Verification items for the finished model (mm, model axes). Face numbers are marked on the shaded views. A direction names the side the tool comes from. Coordinates: 2 decimals unless noted, no trailing zeros. Write each loop counter-clockwise with the first axis right and the second up, starting at its lowest first coordinate (ties: lowest second). Pieces come first, ordered by that corner, then holes. Notation, with made-up numbers: M 45.25,71 L 66.25,71 A12 cw 66.25,88 Z; hole C -34,66.5 d1. An arc over 180 degrees is marked long. One line per item, written item: value.
```python
from build123d import *

# Parameters (mm, degrees)
SKETCH1_W           = 82
SKETCH1_H           = 31
BOSS_EXTRUDE2_DEPTH = 9.525
FILLET2_R           = 2
SKETCH2_R           = 8.119849814
CUT_EXTRUDE1_DEPTH  = 10.525
SKETCH3_W           = 9.5
SKETCH3_H           = 18
CUT_EXTRUDE2_DEPTH  = 10.525
SKETCH5_R           = 2.5
CUT_EXTRUDE4_DEPTH  = 30


with BuildPart() as part:
    # Sketch1 → Boss-Extrude2 (new body)
    with BuildSketch(Plane.XY):
        with Locations((0, 15.5)):
            Rectangle(SKETCH1_W, SKETCH1_H)
    extrude(amount=BOSS_EXTRUDE2_DEPTH)

    # Fillet2
    fillet2_edges = [part.edges().sort_by_distance(p)[0] for p in [
        (-41, 31, 4.7625),
        (41, 31, 4.7625),
        (41, 0, 4.7625),
        (-41, 0, 4.7625),
    ]]
    fillet(fillet2_edges, radius=FILLET2_R)

    # Sketch2 → Cut-Extrude1 (cut, through all)
    with BuildSketch(Plane.XY.offset(9.525)):
        with Locations((0, 15.5)):
            Circle(SKETCH2_R)
    extrude(amount=-CUT_EXTRUDE1_DEPTH, mode=Mode.SUBTRACT)

    # Sketch3 → Cut-Extrude2 (cut, through all)
    with BuildSketch(Plane(origin=(0, 0, 0), x_dir=(-1, 0, 0), z_dir=(0, 0, -1))):
        with Locations((-29.925, 14.5)):
            Rectangle(SKETCH3_W, SKETCH3_H)
    cut_extrude2 = extrude(amount=-CUT_EXTRUDE2_DEPTH, mode=Mode.SUBTRACT)

    # Sketch5 → Cut-Extrude4 (cut)
    with BuildSketch(Plane(origin=(0, 31, 0), x_dir=(1, 0, 0), z_dir=(0, 1, 0))):
        with Locations((-29.925, -4.76)):
            Circle(SKETCH5_R)
    cut_extrude4 = extrude(amount=-CUT_EXTRUDE4_DEPTH, mode=Mode.SUBTRACT)

    # Mirror1: Cut-Extrude2, Cut-Extrude4 across plane
    add(cut_extrude2.mirror(Plane(origin=(0, 0, 0), x_dir=(0, 0, 1), z_dir=(1, 0, 0))), mode=Mode.SUBTRACT)
    add(cut_extrude4.mirror(Plane(origin=(0, 0, 0), x_dir=(0, 0, 1), z_dir=(1, 0, 0))), mode=Mode.SUBTRACT)


solid = part.part
```
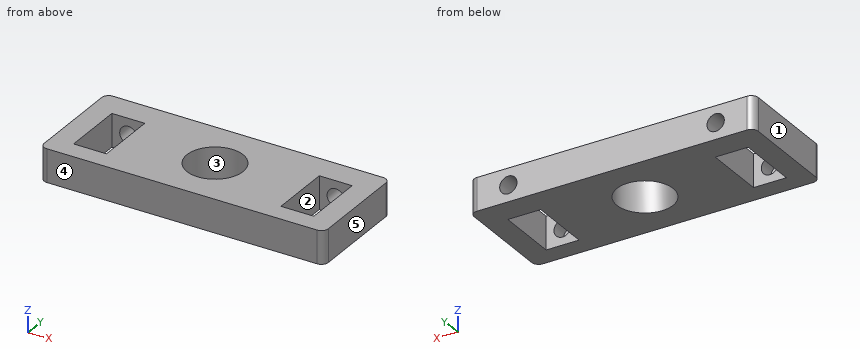
Item 1: Cross-section at B-B, the plane z = 8. Enter the section's corners in (x, y) (3 decimals), and give its area (3 significant figures).
The answers:
outline: M -41,2 A2 ccw -39,0 L 39,0 A2 ccw 41,2 L 41,29 A2 ccw 39,31 L -39,31 A2 ccw -41,29 Z; hole M -34.675,5.5 L -25.175,5.5 L -25.175,23.5 L -34.675,23.5 Z; hole C 0,15.5 d16.24; hole M 25.175,5.5 L 34.675,5.5 L 34.675,23.5 L 25.175,23.5 Z
area: 1,990 mm²
Item 2: Go/stop test with a flat-tipped pin: P1, Ø1.5, axis at x = -30, z = 5.5, coming from the +Y side. Record where the tip stops, or that it passes through.
The answers:
P1: stops at y = 1
Item 3: Cross-section at C-C, the plane x = 0. Enter the section's corners in (y, z) (3 decimals).
The answers:
outline: M 0,0 L 7.38,0 L 7.38,9.525 L 0,9.525 Z; M 23.62,0 L 31,0 L 31,9.525 L 23.62,9.525 Z
Item 4: Scan lines: line 1 (X direction, y = 26.5, z = 4.76) (3 decimals); line 2 (X direction, y = 25.5, z = 2.75); line 3 (X direction, y = 23, z = 2.25) (3 decimals). Record each from-to range of solid material in increasing order.
The answers:
line 1: x = -41 to -32.425, -27.425 to 27.425, 32.425 to 41
line 2: x = -41 to -31.41, -28.44 to 28.44, 31.41 to 41
line 3: x = -41 to -34.675, -25.175 to -3.112, 3.112 to 25.175, 34.675 to 41
Item 5: Access from +Z, -Z, +X, -X, +Y, -Y to the whole of each face (thin tool, end or side, straight path). Record for the marked faces 1 and 2.
The answers:
face 1: +Z, -Z, -X, +Y, -Y
face 2: +Z, -Z
Item 6: Draft check along X on the marked faces 3, 4 and 5. Enter one of: released by +X, released by -X, zero draft, split by the parting line, or undercut.
The answers:
face 3: undercut
face 4: zero draft
face 5: released by +X
Item 7: Cross-section at A-A, the plane y = 15.5. Enter the section's corners in (x, z) (3 decimals), and give its area (3 significant figures).
The answers:
outline: M -41,0 L -34.675,0 L -34.675,9.525 L -41,9.525 Z; M -25.175,0 L -8.12,0 L -8.12,9.525 L -25.175,9.525 Z; M 8.12,0 L 25.175,0 L 25.175,9.525 L 8.12,9.525 Z; M 34.675,0 L 41,0 L 41,9.525 L 34.675,9.525 Z
area: 445 mm²
